Verification items for the finished model (mm, model axes). Give positions to 0.01 mm unless a question says otherwise; leave off trailing zeros. Loops run counter-clockwise (first coordinate to the right, second up) from the corner with the lowest first, then second, coordinate; pieces in that order, holes last. Notation, with made-up numbers: (18, -18) -> (36, -18) arc R24 ccw to (36, 15) -> close; hole circle Ø8 at (79.25, -7.5). An arc over 180 degrees is marked (long way). Answer in a Markdown table with one row per item. Add a question column.
Q1. Section check D-D on x = 43. Enter the section's corners in (y, z).
Q2. Section check A-A on y = 40. Enter the section's corners in (x, z), and give its area (3 significant figures).
Q3. Section check B-B on x = 10. Enter the section's corners in (y, z).
Q4. Gauge pin test, flat end, axial feed: P1, Ø2.5, axis at x = 32, z = 1.5, coming from the -Y side. Record the tip position at first contact, or that the pin passes through.
Q5. Material ranges on probe 1 along Y at (x, z) = (10, 3.65); probe 2 along Y at (x, z) = (9.5, 1.5); probe 3 along X at (y, z) = (38, 0.7), recorded low to high.
Q6. Section check C-C on z = 3.4. Enter the section's corners in (x, y).
Autodesk Inventor part; units mm, degrees
ref_plane "YZ Plane" through (0, 0, 0) normal (1, 0, 0) x (0, 1, 0)
ref_plane "XZ Plane" through (0, 0, 0) normal (0, 1, 0) x (-1, 0, 0)
ref_plane "XY Plane" through (0, 0, 0) normal (0, 0, 1) x (1, 0, 0)
sketch "Sketch1" plane through (0, 0, 0) normal (0, 0, 1) x (1, 0, 0)
  line L0 (0, 0) -> (120, 0)
  line L1 (120, 0) -> (120, 75)
  line L2 (120, 75) -> (0, 75)
  line L3 (0, 75) -> (0, 0)
  circle A0 centre (10, 40) radius 2.5
  dimension "d0" = 120
  dimension "d1" = 75
  dimension "d2" = 5
  dimension "d3" = 10
  dimension "d4" = 35
extrude "Extrusion1" add sketch "Sketch1" along normal blind 5
sketch "Sketch2" plane through (0, 0, 5) normal (0, 0, 1) x (1, 0, 0)
  line L0 (0, 0) -> (120, 0)
  line L1 (24, 0) -> (48, 0)
  line L2 (48, 0) -> (48, 5)
  line L3 (48, 5) -> (24, 5)
  line L4 (24, 5) -> (24, 0)
  line L5 (72, 0) -> (96, 0)
  line L6 (96, 0) -> (96, 5)
  line L7 (96, 5) -> (72, 5)
  line L8 (72, 5) -> (72, 0)
  line L9 (0, 75) -> (0, 0)
  dimension "d7" = 24
  dimension "d8" = 5
  dimension "d9" = 24
  dimension "d10" = 5
  dimension "d11" = 24
  dimension "d12" = 24
extrude "Extrusion2" cut sketch "Sketch2" against normal blind 5
sketch "Sketch3" plane through (0, 0, 5) normal (0, 0, 1) x (1, 0, 0)
  line L0 (38.7826, 73.4019) -> (98.6345, 73.4019) construction
  line L1 (98.6345, 73.4019) -> (98.6345, 53.9975) construction
  line L2 (98.6345, 53.9975) -> (38.7826, 53.9975) construction
  line L3 (38.7826, 53.9975) -> (38.7826, 73.4019) construction
  point P0 (0, 0)
sketch "Sketch4" plane through (48, 0, 0) normal (0, -1, 0) x (1, 0, 0)
  line L0 (2.1203, 4.645) -> (24.7173, 4.645) construction
  line L1 (24.7173, 4.645) -> (24.7173, 0.4931) construction
  line L2 (24.7173, 0.4931) -> (2.1203, 0.4931) construction
  line L3 (2.1203, 0.4931) -> (2.1203, 4.645) construction
  point P0 (-48, 0)
sketch "Sketch5" plane through (0, 0, 0) normal (0, 0, -1) x (-1, 0, 0)
  line L0 (-77.429, 73.1669) -> (18.9429, 73.1669) construction
  line L1 (18.9429, 73.1669) -> (18.9429, 43.3318) construction
  line L2 (18.9429, 43.3318) -> (-77.429, 43.3318) construction
  line L3 (-77.429, 43.3318) -> (-77.429, 73.1669) construction
  point P0 (0, 0)
properties part number "SpurGearMount"
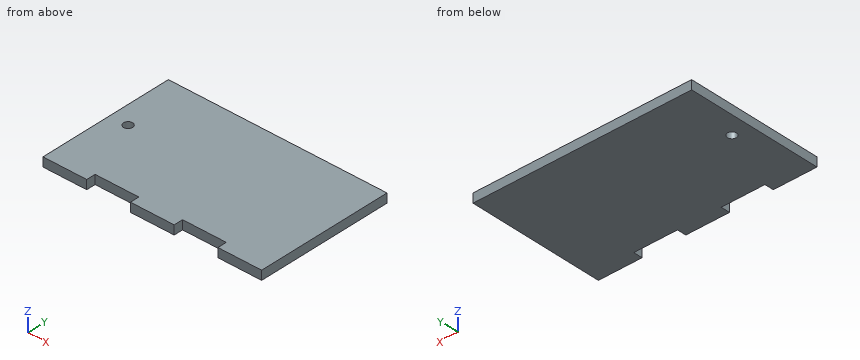
Taken from the geometry:
| question | item | result |
|---|---|---|
| 1 | outline | (5, 0) -> (75, 0) -> (75, 5) -> (5, 5) -> close |
| 2 | outline | (0, 0) -> (7.5, 0) -> (7.5, 5) -> (0, 5) -> close; (12.5, 0) -> (120, 0) -> (120, 5) -> (12.5, 5) -> close |
| 2 | area | 575 mm² |
| 3 | outline | (0, 0) -> (37.5, 0) -> (37.5, 5) -> (0, 5) -> close; (42.5, 0) -> (75, 0) -> (75, 5) -> (42.5, 5) -> close |
| 4 | P1 | stops at y = 5 |
| 5 | probe 1 | y = 0 to 37.5, 42.5 to 75 |
| 5 | probe 2 | y = 0 to 37.55, 42.45 to 75 |
| 5 | probe 3 | x = 0 to 8.5, 11.5 to 120 |
| 6 | outline | (0, 0) -> (24, 0) -> (24, 5) -> (48, 5) -> (48, 0) -> (72, 0) -> (72, 5) -> (96, 5) -> (96, 0) -> (120, 0) -> (120, 75) -> (0, 75) -> close; hole circle Ø5 at (10, 40) |
